Part model, mm, in its own coordinate system. A direction names the side the tool comes from. Give positions to 0.01 mm unless a question says otherwise; leave off trailing zeros. Write each loop counter-clockwise with the first axis right and the second up, starting at its lowest first coordinate (ties: lowest second). Pieces come first, ordered by that corner, then holes.
```python
from build123d import *

# Parameters (mm, degrees)
F1_DEPTH      = 40
F1_DEPTH_BACK = 1.2
F0_W          = 8
F0_H          = 3
F0_W_2        = 18.5
F0_H_2        = 1.2
F2_DEPTH      = 1.2
F3_DEPTH      = 25


with BuildPart() as f1:
    # F0 (on Top) → F1 (new body, two sides)
    with BuildSketch(Plane.XY) as f1_sk:
        with BuildLine():
            Line((10.45, -8.1), (10.45, 8.1))
            ThreePointArc((10.45, 8.1), (9.952082, 9.302082), (8.75, 9.8))
            Line((8.75, 9.8), (-8.75, 9.8))
            ThreePointArc((-8.75, 9.8), (-9.952082, 9.302082), (-10.45, 8.1))
            Line((-10.45, 8.1), (-10.45, -8.1))
            ThreePointArc((-10.45, -8.1), (-9.952082, -9.302082), (-8.75, -9.8))
            Line((-8.75, -9.8), (8.75, -9.8))
            ThreePointArc((8.75, -9.8), (9.952082, -9.302082), (10.45, -8.1))
        make_face()
        with BuildLine():
            ThreePointArc((9.25, -8.1), (9.103553, -8.453553), (8.75, -8.6))
            Line((8.75, -8.6), (-8.75, -8.6))
            ThreePointArc((-8.75, -8.6), (-9.103553, -8.453553), (-9.25, -8.1))
            Line((-9.25, -8.1), (-9.25, -0.6))
            Line((-9.25, -0.6), (-9.25, 0.6))
            Line((-9.25, 0.6), (-9.25, 8.1))
            ThreePointArc((-9.25, 8.1), (-9.103553, 8.453553), (-8.75, 8.6))
            Line((-8.75, 8.6), (8.75, 8.6))
            ThreePointArc((8.75, 8.6), (9.103553, 8.453553), (9.25, 8.1))
            Line((9.25, 8.1), (9.25, 0.6))
            Line((9.25, 0.6), (9.25, -0.6))
            Line((9.25, -0.6), (9.25, -8.1))
        make_face(mode=Mode.SUBTRACT)
    extrude(amount=F1_DEPTH)
    extrude(f1_sk.sketch, amount=-F1_DEPTH_BACK)

    # F0 (on Top) → F2 (join)
    with BuildSketch(Plane.XY):
        with BuildLine():
            Line((-9.25, 0.6), (9.25, 0.6))
            Line((9.25, 0.6), (9.25, 8.1))
            ThreePointArc((9.25, 8.1), (9.103553, 8.453553), (8.75, 8.6))
            Line((8.75, 8.6), (-8.75, 8.6))
            ThreePointArc((-8.75, 8.6), (-9.103553, 8.453553), (-9.25, 8.1))
            Line((-9.25, 8.1), (-9.25, 0.6))
        make_face()
        with Locations((-0.65, 4.7)):
            Rectangle(F0_W, F0_H, mode=Mode.SUBTRACT)
        Rectangle(F0_W_2, F0_H_2)
        with BuildLine():
            Line((-8.75, -8.6), (8.75, -8.6))
            ThreePointArc((8.75, -8.6), (9.103553, -8.453553), (9.25, -8.1))
            Line((9.25, -8.1), (9.25, -0.6))
            Line((9.25, -0.6), (-9.25, -0.6))
            Line((-9.25, -0.6), (-9.25, -8.1))
            ThreePointArc((-9.25, -8.1), (-9.103553, -8.453553), (-8.75, -8.6))
        make_face()
        with Locations((-0.65, -4.5)):
            Rectangle(F0_W, F0_H, mode=Mode.SUBTRACT)
    extrude(amount=-F2_DEPTH)

    # F0 (on Top) → F3 (join)
    with BuildSketch(Plane.XY):
        Rectangle(F0_W_2, F0_H_2)
    extrude(amount=F3_DEPTH)


solid = f1.part
```
1) Pin check, flat tips, straight feed: pin 1 Ø0.6 at (x, y) = (-2.5, 0) entering from +Z; pin 2 Ø6.5 at (x, y) = (-0.5, 5) entering from +Z; pin 3 Ø6 at (x, y) = (-8, 6.5) entering from +Z. Stop position of each tip, or through.
Answers follow:
pin 1: stops at z = 25
pin 2: stops at z = 0
pin 3: stops at z = 40
2) Saw through at A-A, the plane z = 34.5. Write the cut outline in (x, y), then the cut area to 3 significant figures.
Answers follow:
outline: (-10.45, -8.1) arc R1.7 ccw to (-8.75, -9.8) - (8.75, -9.8) arc R1.7 ccw to (10.45, -8.1) - (10.45, 8.1) arc R1.7 ccw to (8.75, 9.8) - (-8.75, 9.8) arc R1.7 ccw to (-10.45, 8.1) - close; hole (-9.25, -8.1) arc R0.5 ccw to (-8.75, -8.6) - (8.75, -8.6) arc R0.5 ccw to (9.25, -8.1) - (9.25, 8.1) arc R0.5 ccw to (8.75, 8.6) - (-8.75, 8.6) arc R0.5 ccw to (-9.25, 8.1) - close
area: 89.2 mm2
3) Saw through at C-C, the plane x = -2.25. Write the cut outline in (y, z), then the cut area to 3 significant figures.
Answers follow:
outline: (-9.8, -1.2) - (-6, -1.2) - (-6, 0) - (-8.6, 0) - (-8.6, 40) - (-9.8, 40) - close; (-3, -1.2) - (3.2, -1.2) - (3.2, 0) - (0.6, 0) - (0.6, 25) - (-0.6, 25) - (-0.6, 0) - (-3, 0) - close; (6.2, -1.2) - (9.8, -1.2) - (9.8, 40) - (8.6, 40) - (8.6, 0) - (6.2, 0) - close
area: 142 mm2
4) Saw through at D-D, the plane z = 15. Write the cut outline in (x, y).
Answers follow:
outline: (-10.45, -8.1) arc R1.7 ccw to (-8.75, -9.8) - (8.75, -9.8) arc R1.7 ccw to (10.45, -8.1) - (10.45, 8.1) arc R1.7 ccw to (8.75, 9.8) - (-8.75, 9.8) arc R1.7 ccw to (-10.45, 8.1) - close; hole (-9.25, -8.1) arc R0.5 ccw to (-8.75, -8.6) - (8.75, -8.6) arc R0.5 ccw to (9.25, -8.1) - (9.25, -0.6) - (-9.25, -0.6) - close; hole (-9.25, 0.6) - (9.25, 0.6) - (9.25, 8.1) arc R0.5 ccw to (8.75, 8.6) - (-8.75, 8.6) arc R0.5 ccw to (-9.25, 8.1) - close
5) Wall check: L1, parallel to Y at x = 0, z = 1; L2, parallel to X at y = -2.25, z = 17.5; L3, parallel to Z at x = -5.5, y = -4.25. Give the ranges that are in metal, low to high.
Answers follow:
L1: y = -9.8 to -8.6, -0.6 to 0.6, 8.6 to 9.8
L2: x = -10.45 to -9.25, 9.25 to 10.45
L3: z = -1.2 to 0
6) Saw through at B-B, the plane y = 5. Write the cut outline in (x, z), then the cut area to 3 significant figures.
Answers follow:
outline: (-10.45, -1.2) - (-4.65, -1.2) - (-4.65, 0) - (-9.25, 0) - (-9.25, 40) - (-10.45, 40) - close; (3.35, -1.2) - (10.45, -1.2) - (10.45, 40) - (9.25, 40) - (9.25, 0) - (3.35, 0) - close
area: 111 mm2
7) 3-axis set-ups, long thin cutter, end or side, ignore diameter. For faces 4 (the face through (-9.965, -9.289, 19.688)), 5 (the face through (9.25, 2, 20)), 6 (the face through (3.35, -5, -1)): which of +Z, -Z, +X, -X, +Y, -Y reach the whole face in a straight line?
Answers follow:
face 4: +Z, -Z, -X, -Y
face 5: +Z
face 6: +Z, -Z
8) Two-plate mould, pull along Z, no slides. Class faces 1 (the face through (-0.1, -6.3, 0)), 2 (the face through (0, 0, -1.2)), 3 (the face through (-1, 3.2, -1)): +Z half, -Z half, draft (parallel to the pull), parting line (faces both ways), or undercut.
Answers follow:
face 1: +Z half
face 2: -Z half
face 3: draft
